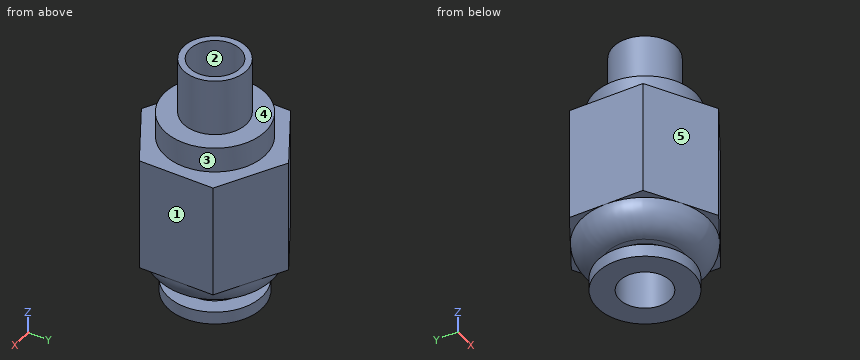
from build123d import *

# Parameters (mm, degrees)
EXTRUDE_1_DEPTH     = 9
SKETCH_2_R          = 4
EXTRUDE_2_DEPTH     = 2
SKETCH_3_R          = 2.5
EXTRUDE_3_DEPTH     = 4.5
EXTRUDE_START       = 1
SKETCH_5_R          = 2.5
EXTRUDE_4_DEPTH     = 1
SKETCH_6_R          = 3.75
EXTRUDE_5_DEPTH     = 1
SKETCH_7_R          = 2
CUT_EXTRUDE_1_DEPTH = 21.942381272


with BuildPart() as part:
    # 草图1 → 凸台-拉伸1 (new body)
    with BuildSketch(Plane.XY):
        Polygon((5, 2.886751346), (0, 5.773502692), (-5, 2.886751346), (-5, -2.886751346), (0, -5.773502692), (5, -2.886751346), align=None)
    extrude(amount=EXTRUDE_1_DEPTH)

    # 草图2 → 凸台-拉伸2 (add)
    with BuildSketch(Plane.XY.offset(9)):
        Circle(SKETCH_2_R)
    extrude(amount=EXTRUDE_2_DEPTH)

    # 草图3 → 凸台-拉伸3 (add)
    with BuildSketch(Plane.XY.offset(11)):
        Circle(SKETCH_3_R)
    extrude(amount=EXTRUDE_3_DEPTH)

    # 草图4 → 旋转1 (revolve)
    with BuildSketch(Plane(origin=(0, 0, 0), x_dir=(1, 0, 0), z_dir=(0, 1, 0))):
        with BuildLine():
            Line((0, 0), (0, 2))
            Line((0, 2), (3, 2))
            ThreePointArc((3, 2), (4.414213562, 1.414213562), (5, 0))
            Line((5, 0), (0, 0))
        make_face()
    revolve(axis=Axis((0, 0, 0), (0, 0, -1)))

    # 草图5 → 凸台-拉伸4 (add)
    with BuildSketch(Plane(origin=(0, 0, -2), x_dir=(-1, 0, 0), z_dir=(0, 0, -1)).offset(EXTRUDE_START)):
        with Locations(Location((0, 0, 0), (0, 0, 180))):
            Circle(SKETCH_5_R)
    extrude(amount=-EXTRUDE_4_DEPTH)

    # 草图6 → 凸台-拉伸5 (add)
    with BuildSketch(Plane(origin=(0, 0, -3), x_dir=(-1, 0, 0), z_dir=(0, 0, -1))):
        Circle(SKETCH_6_R)
    extrude(amount=EXTRUDE_5_DEPTH)

    # 草图7 → 切除-拉伸1 (cut, through all)
    with BuildSketch(Plane(origin=(0, 0, -4), x_dir=(-1, 0, 0), z_dir=(0, 0, -1))):
        Circle(SKETCH_7_R)
    extrude(amount=-CUT_EXTRUDE_1_DEPTH, mode=Mode.SUBTRACT)


solid = part.part
Can you work these out from the model? Positions are in its coordinate system, mm. Face numbers are marked on the shaded views. A direction names the side the tool comes from. Coordinates: 2 decimals unless noted, no trailing zeros. Loops run counter-clockwise (first coordinate to the right, second up) from the corner with the lowest first, then second, coordinate; pieces in that order, holes last. Notation, with made-up numbers: M 40.5,67.5 L 68.5,67.5 A33 ccw 68.5,105.5 Z; hole C 25.5,82.5 d9. An arc over 180 degrees is marked long. Return JSON: item names as keys, results as strings. Group by question number.
Item 1: If I drill on L1, parallel to Y at x = -2.5, z = 2.25; L2, parallel to Y at x = -1.25, z = 13.75; L3, parallel to Y at x = 0.25, z = 12, over which ranges is the centre line in solid material (lowest first)? Write a range as from..to.
Item 2: I'm going to push flat-ended pins straight in: pin 1 Ø6 at (x, z) = (0, 4.5) entering from +Y; pin 2 Ø0.8 at (x, y) = (-4, 1.5) entering from -Z; pin 3 Ø0.7 at (x, y) = (0.5, -5) entering from -Z. Where does each tip first touch, or does it pass through?
Item 3: On a 3-axis mill with a long thin cutter (end or side, diameter ignored), from which of +Z, -Z, +X, -X, +Y, -Y can I reach the whole of each face in a straight line? I mean the marked faces 4 and 5. Say none if no direction works.
Item 4: Thinking about a two-plate mould opening in Y: for the marked faces 1, 2 and 3, which applies, released by +Y, released by -Y, zero draft, split by the parting line, or undercut?
Item 5: Imagine slicing it at A-A (z = 3). Please give me the cut outline in (x, y), and give its area (3 significant figures).
Verdict:
{
 "1": {"L1": "y = -4.33..4.33", "L2": "y = -2.17..-1.56, 1.56..2.17", "L3": "y = -2.49..-1.98, 1.98..2.49"},
 "2": {"pin 1": "stops at y = 5.77", "pin 2": "stops at z = -1.8", "pin 3": "stops at z = -1.09"},
 "3": {"face 4": "+Z", "face 5": "+Z, -Z, -X, -Y"},
 "4": {"face 1": "zero draft", "face 2": "undercut", "face 3": "split by the parting line"},
 "5": {"outline": "M -5,-2.89 L 0,-5.77 L 5,-2.89 L 5,2.89 L 0,5.77 L -5,2.89 Z; hole C 0,0 d4", "area": "74.0 mm^2"}
}
